from build123d import *

# Parameters (mm, degrees)
F1_DEPTH = 6
F3_DEPTH = 6.001


with BuildPart() as f1:
    # F0 (on Front) → F1 (new body)
    with BuildSketch(Plane.XZ):
        with BuildLine():
            Line((-182.5, 23), (-189, 23))
            Line((-189, 23), (-189, -23))
            Line((-189, -23), (189, -23))
            Line((189, -23), (189, 23))
            Line((189, 23), (182.5, 23))
            ThreePointArc((182.5, 23), (139.651429, -11), (96.802859, 23))
            Line((96.802859, 23), (89.399047, 23))
            ThreePointArc((89.399047, 23), (46.550476, -11), (3.701906, 23))
            Line((3.701906, 23), (-3.701906, 23))
            ThreePointArc((-3.701906, 23), (-46.550476, -11), (-89.399047, 23))
            Line((-89.399047, 23), (-96.802859, 23))
            ThreePointArc((-96.802859, 23), (-139.651429, -11), (-182.5, 23))
        make_face()
    extrude(amount=F1_DEPTH)

    # F2 (on face) → F3 (cut, through all)
    with BuildSketch(Plane.XZ.offset(6)):
        Polygon((189, -1.6), (189, 1.6), (182.5, 1.6), (182.5, 3.1), (180, 3.1), (180, 1.6), (177, 1.6), (177, -1.6), (180, -1.6), (180, -3.1), (182.5, -3.1), (182.5, -1.6), align=None)
        Polygon((-177, -1.6), (-177, 1.6), (-180, 1.6), (-180, 3.1), (-182.5, 3.1), (-182.5, 1.6), (-189, 1.6), (-189, -1.6), (-182.5, -1.6), (-182.5, -3.1), (-180, -3.1), (-180, -1.6), align=None)
    extrude(amount=-F3_DEPTH, mode=Mode.SUBTRACT)


solid = f1.part
Verification items for the finished model (mm, model axes). A direction names the side the tool comes from. Give positions to 0.01 mm unless a question says otherwise; leave off trailing zeros. Write each loop counter-clockwise with the first axis right and the second up, starting at its lowest first coordinate (ties: lowest second). Pieces come first, ordered by that corner, then holes. Notation, with made-up numbers: M 11,53.5 L 63,53.5 A27 ccw 63,83.5 Z; hole C 61.5,73.25 d3. An arc over 180 degrees is marked long. Write item = value, one per line.
(1) Access from +Z, -Z, +X, -X, +Y, -Y to the whole of each face (thin tool, end or side, straight path). Record for faces 1 (the face through (-186, -3, -1.6)), 2 (the face through (47.377, -2.958, -10.992)), 3 (the face through (186, -3, -1.6)).
Found:
face_1 = -X, +Y, -Y
face_2 = +Z, +Y, -Y
face_3 = +X, +Y, -Y
(2) Sectioned sample at B-B (x = -52.5). Record the cut outline in (y, z).
Found:
outline = M -6,-23 L 0,-23 L 0,-10.6 L -6,-10.6 Z
(3) Sectioned sample at A-A (z = 15.5). Record the cut outline in (x, y).
Found:
outline = M -189,-6 L -180.02,-6 L -180.02,0 L -189,0 Z; M -99.28,-6 L -86.92,-6 L -86.92,0 L -99.28,0 Z; M -6.18,-6 L 6.18,-6 L 6.18,0 L -6.18,0 Z; M 86.92,-6 L 99.28,-6 L 99.28,0 L 86.92,0 Z; M 180.02,-6 L 189,-6 L 189,0 L 180.02,0 Z
(4) Material ranges on line 1 (X direction, y = -4.15, z = 4); line 2 (X direction, y = -3.25, z = 7.5); line 3 (Z direction, x = 138, y = -0.3), recorded low to high.
Found:
line_1 = -189 to -172.74, -106.56 to -79.64, -13.46 to 13.46, 79.64 to 106.56, 172.74 to 189
line_2 = -189 to -175.51, -103.79 to -82.41, -10.69 to 10.69, 82.41 to 103.79, 175.51 to 189
line_3 = -23 to -10.97
(5) Go/stop test with flat-tipped pins: pin 1 Ø1.5 at (x, y) = (179, -3) entering from +Z; pin 2 Ø1.5 at (x, y) = (-178.5, -4.5) entering from +Z; pin 3 Ø1 at (y, z) = (-2.5, 0.5) entering from -X. Record where each tip stops, or that it passes through.
Found:
pin_1 = 14.89
pin_2 = 13.82
pin_3 = -177
(6) Sectioned sample at C-C (x = 71.5). Record the cut outline in (y, z).
Found:
outline = M -6,-23 L 0,-23 L 0,-3.24 L -6,-3.24 Z
(7) Draft check along Z on faces 4 (the face through (-189, -3, 12)), 5 (the face through (-93, -3, 23)), 6 (the face through (186, -3, 1.6)). Enter one of: released by +Z, released by -Z, zero draft, split by the parting line, or undercut.
Found:
face_4 = zero draft
face_5 = released by +Z
face_6 = undercut
